Autodesk Inventor part; units mm, degrees
ref_plane "YZ Plane" through (0, 0, 0) normal (1, 0, 0) x (0, 1, 0)
ref_plane "XZ Plane" through (0, 0, 0) normal (0, 1, 0) x (-1, 0, 0)
ref_plane "XY Plane" through (0, 0, 0) normal (0, 0, 1) x (1, 0, 0)
sketch "スケッチ1" plane through (0, 0, 0) normal (0, 1, 0) x (-1, 0, 0)
  line L0 (-12.5, -2) -> (12.5, -2)
  line L1 (12.5, -2) -> (12.5, 2)
  line L2 (12.5, 2) -> (-12.5, 2)
  line L3 (-12.5, 2) -> (-12.5, -2)
  line L4 (-12.5, -2) -> (12.5, 2) construction
  line L5 (12.5, -2) -> (-12.5, 2) construction
  point P0 (0, 0)
  dimension "d0" = 25
  dimension "d1" = 4
extrude "押し出し1" add sketch "スケッチ1" along normal mid plane 5
sketch "スケッチ2" plane through (0, 0, 0) normal (0, 0, 1) x (1, 0, 0)
  circle A0 centre (-10.5, 0) radius 1.25
  line L0 (-12.5, -2.5) -> (-12.5, 2.5)
  circle A1 centre (10.5, 0) radius 1.25
  line L1 (12.5, -2.5) -> (12.5, 2.5)
  point P0 (0, 0)
  dimension "d4" = 2.5
  dimension "d5" = 2
  dimension "d14" = 2.5
  dimension "d15" = 2
extrude "押し出し2" cut sketch "スケッチ2" along normal mid plane 5 contours A0
chamfer "面取り1" distance 2 angle 45 1 edges at (-12.5, 2.5, 0)
chamfer "面取り2" distance 2 angle 45 1 edges at (-12.5, -2.5, 0)
sketch "スケッチ3" plane through (0, 0, 0) normal (0, 0, 1) x (1, 0, 0)
  circle A0 centre (10.5, 0) radius 1.25
  line L0 (12.5, -2.5) -> (12.5, 2.5)
  point P0 (0, 0)
  dimension "d16" = 2.5
  dimension "d17" = 2
extrude "押し出し3" cut sketch "スケッチ3" along normal mid plane 5
chamfer "面取り3" distance 2 angle 45 1 edges at (12.5, 2.5, 0)
chamfer "面取り4" distance 2 angle 45 1 edges at (12.5, -2.5, 0)
sketch "スケッチ4" plane through (0, -2.5, 0) normal (0, -1, 0) x (1, 0, 0)
  line L0 (-12.5, -2) -> (-12.5, 2)
  line L1 (-12.5, 0) -> (-8.5, 0)
  line L2 (-8.5, 0) -> (-8.5, 2)
  line L3 (-8.5, 2) -> (-12.5, 2)
  line L4 (-12.5, 2) -> (-12.5, 0)
  point P0 (0, 0)
  dimension "d26" = 4
extrude "押し出し4" cut sketch "スケッチ4" against normal blind 10
properties part number "promo_arm1'"
Source: CAD feature listing. Evaluate the final solid. Frame: model axes, mm. A direction names the side the tool comes from. Coordinates: 2 decimals unless noted, no trailing zeros. Write each loop counter-clockwise with the first axis right and the second up, starting at its lowest first coordinate (ties: lowest second). Pieces come first, ordered by that corner, then holes. Notation, with made-up numbers: (69, 86) -> (97, 86) arc R31 cw to (97, 122) -> close; hole circle Ø1 at (-12.75, 86.25). An arc over 180 degrees is marked (long way). Return JSON: item names as keys, results as strings. Group by question number.
1) Section query C-C, the plane y = 2.1. Return loops of the section in (x, z).
2) Set-up query: faces 4 (the face through (-9, 0, 0)), 5 (the face through (9.25, 0.05, 0.03)). Return all of +Z, -Z, +X, -X, +Y, -Y with unobstructed straight access to the full face (end or side cutting, diameter ignored); none if empty.
3) Mould query, pull axis X, two halves, no side actions, for faces 1 (the face through (-11.75, 0.05, -0.99)), 2 (the face through (-8.5, 0, 1)), 3 (the face through (0, 2.5, 0)). Classes: +X half, -X half, draft (parallel to the pull), parting line (faces both ways), or undercut.
4) Section query D-D, the plane y = -0.95. Return loops of the section in (x, z), plus the area to 3 significant figures.
5) Section query B-B, the plane z = 1. Return loops of the section in (x, y).
6) Section query A-A, the plane y = 0. Return loops of the section in (x, z).
7) Ray query, line 1 along X through (y, z) = (0.05, -1.2); line 2 along Y through (x, z) = (-11.5, -0.9); line 3 along X through (y, z) = (0.65, 0.05). Return the intervals inside material, ascending.
8) Contact query for a flat-ended pin moving along its axis: P1, Ø3, axis at x = 10.5, y = 0, coming from the +Z side. Output: stop coordinate, or through.
From the geometry:
{
 "1": {"outline": "(-10.9, -2) -> (10.9, -2) -> (10.9, 2) -> (-8.5, 2) -> (-8.5, 0) -> (-10.9, 0) -> close"},
 "2": {"face 4": "+Z, -X, +Y, -Y", "face 5": "+Z, -Z"},
 "3": {"face 1": "undercut", "face 2": "-X half", "face 3": "draft"},
 "4": {"outline": "(-12.05, -2) -> (-11.31, -2) -> (-11.31, 0) -> (-12.05, 0) -> close; (-9.69, -2) -> (9.69, -2) -> (9.69, 2) -> (-8.5, 2) -> (-8.5, 0) -> (-9.69, 0) -> close; (11.31, -2) -> (12.05, -2) -> (12.05, 2) -> (11.31, 2) -> close", "area": "79.6 mm²"},
 "5": {"outline": "(-8.5, -2.5) -> (10.5, -2.5) -> (12.5, -0.5) -> (12.5, 0.5) -> (10.5, 2.5) -> (-8.5, 2.5) -> close; hole circle Ø2.5 at (10.5, 0)"},
 "6": {"outline": "(-12.5, -2) -> (-11.75, -2) -> (-11.75, 0) -> (-12.5, 0) -> close; (-9.25, -2) -> (9.25, -2) -> (9.25, 2) -> (-8.5, 2) -> (-8.5, 0) -> (-9.25, 0) -> close; (11.75, -2) -> (12.5, -2) -> (12.5, 2) -> (11.75, 2) -> close"},
 "7": {"line 1": "-12.5 to -11.75, -9.25 to 9.25, 11.75 to 12.5", "line 2": "-1.5 to -0.75, 0.75 to 1.5", "line 3": "-8.5 to 9.43, 11.57 to 12.35"},
 "8": {"P1": "z = 2"}
}
